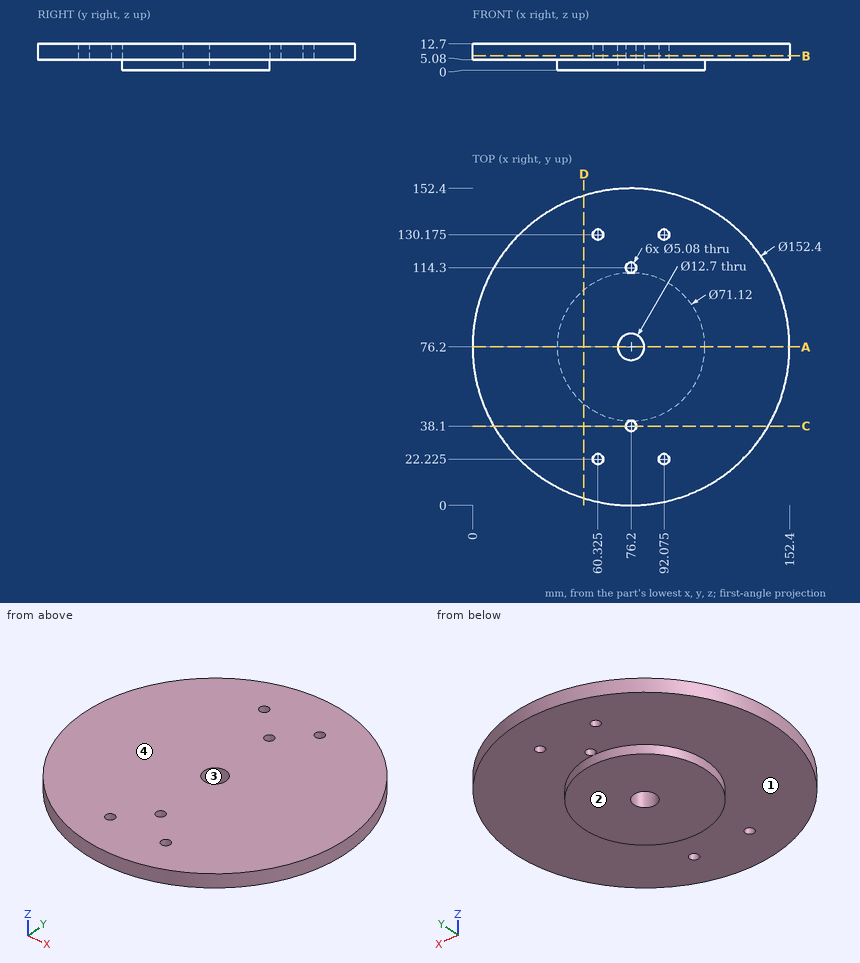
Can you work these out from the drawing? Everything is in mm from the part's minimum corner. A direction names the side the tool comes from. Round coordinates to 2 decimals unless told otherwise and drop trailing zeros. Write each loop counter-clockwise with the first axis right and the second up, starting at its lowest first coordinate (ties: lowest second). Pieces come first, ordered by that corner, then holes. Notation, with made-up numbers: M 88,80 L 123,80 A14 ccw 123,104 Z; hole C 14,88 d5. An arc over 180 degrees is marked long. Use a Markdown table: item, result.
Item 1: I want a section at B-B (z = 7). List the corners of the cut face in (x, y) for me (3 decimals).
Found:
| item | result |
|---|---|
| outline | C 76.2,76.2 d152.4; hole C 60.325,22.225 d5.08; hole C 60.325,130.175 d5.08; hole C 76.2,76.2 d12.7; hole C 76.2,38.1 d5.08; hole C 76.2,114.3 d5.08; hole C 92.075,22.225 d5.08; hole C 92.075,130.175 d5.08 |
Item 2: Which directions (+Z, -Z, +X, -X, +Y, -Y) give clear straight access to the entire face, cutting with the end or side of a thin tool? Please do the marked faces 1 and 2.
Found:
| item | result |
|---|---|
| face 1 | -Z |
| face 2 | -Z, +X, -X, +Y, -Y |
Item 3: I want a section at A-A (y = 76.2). List the corners of the cut face in (x, z) for me, and give its area (3 significant figures).
Found:
| item | result |
|---|---|
| outline | M 0,5.08 L 40.64,5.08 L 40.64,0 L 69.85,0 L 69.85,12.7 L 0,12.7 Z; M 82.55,0 L 111.76,0 L 111.76,5.08 L 152.4,5.08 L 152.4,12.7 L 82.55,12.7 Z |
| area | 1,360 mm2 |
Item 4: I want a section at D-D (x = 53.5). List the corners of the cut face in (y, z) for me.
Found:
| item | result |
|---|---|
| outline | M 3.46,5.08 L 48.83,5.08 L 48.83,0 L 103.57,0 L 103.57,5.08 L 148.94,5.08 L 148.94,12.7 L 3.46,12.7 Z |
Item 5: We'd pull the mould along Y, two halves only. Please class the marked faces 3 and 4: released by +Y, released by -Y, zero draft, split by the parting line, or undercut.
Found:
| item | result |
|---|---|
| face 3 | undercut |
| face 4 | zero draft |
Item 6: For pin 1 Ø2 at (x, z) = (74.5, 2.5) entering from +Y; pin 2 Ø6 at (x, z) = (87.5, 9.5) entering from -Y; pin 3 Ø8 at (x, y) = (60.325, 22.225) entering from -Z, each with a flat end and sliding along its axis, tell me the tip position at first contact or that it passes through.
Found:
| item | result |
|---|---|
| pin 1 | stops at y = 111.75 |
| pin 2 | stops at y = 0.45 |
| pin 3 | stops at z = 5.08 |
Item 7: If I drill on line 1 along Y through (x, z) = (76.2, 10.5); line 2 along Y through (x, z) = (76.5, 0.5); line 3 along X through (y, z) = (76.2, 2.5), over which ranges is the centre line in solid material (lowest first)? Write a range as [from, to].
Found:
| item | result |
|---|---|
| line 1 | y = [0, 35.56], [40.64, 69.85], [82.55, 111.76], [116.84, 152.4] |
| line 2 | y = [40.64, 69.86], [82.54, 111.76] |
| line 3 | x = [40.64, 69.85], [82.55, 111.76] |
Item 8: I want a section at C-C (y = 38.1). List the corners of the cut face in (x, z) for me.
Found:
| item | result |
|---|---|
| outline | M 10.21,5.08 L 73.66,5.08 L 73.66,12.7 L 10.21,12.7 Z; M 78.74,5.08 L 142.19,5.08 L 142.19,12.7 L 78.74,12.7 Z |
